```python
from build123d import *

# Parameters (mm, degrees)
SKETCH1_W           = 20
SKETCH1_H           = 18
BOSS_EXTRUDE1_DEPTH = 8
SKETCH2_W           = 18
SKETCH2_H           = 5
CUT_EXTRUDE1_DEPTH  = 6
SKETCH4_W           = 18
SKETCH4_H           = 5
CUT_EXTRUDE2_DEPTH  = 13
SKETCH5_W           = 18
SKETCH5_H           = 4
CUT_EXTRUDE3_DEPTH  = 4


with BuildPart() as part:
    # Sketch1 → Boss-Extrude1 (new body)
    with BuildSketch(Plane.XY):
        Rectangle(SKETCH1_W, SKETCH1_H)
    extrude(amount=BOSS_EXTRUDE1_DEPTH)

    # Sketch2 → Cut-Extrude1 (cut)
    with BuildSketch(Plane.XY.offset(8)):
        with Locations((0, -5.5)):
            Rectangle(SKETCH2_W, SKETCH2_H)
    extrude(amount=-CUT_EXTRUDE1_DEPTH, mode=Mode.SUBTRACT)

    # Sketch4 → Cut-Extrude2 (cut)
    with BuildSketch(Plane.XZ.offset(3)):
        with Locations((0, 4.5)):
            Rectangle(SKETCH4_W, SKETCH4_H)
    extrude(amount=-CUT_EXTRUDE2_DEPTH, mode=Mode.SUBTRACT)

    # Sketch5 → Cut-Extrude3 (cut)
    with BuildSketch(Plane(origin=(0, 0, 0), x_dir=(-1, 0, 0), z_dir=(0, 0, -1))):
        with Locations((0, 7)):
            Rectangle(SKETCH5_W, SKETCH5_H)
    extrude(amount=-CUT_EXTRUDE3_DEPTH, mode=Mode.SUBTRACT)


solid = part.part
```
The model under review builds one solid part; all positions refer to its coordinate system, in mm. A direction names the side the tool comes from. Round coordinates to 2 decimals unless told otherwise and drop trailing zeros. Order: outer loops, then holes, each group sorted by start corner. A loop starts at its lowest first (then second) coordinate and runs counter-clockwise, first axis right, second up.
Item 1: To check wall thickness, follow probe 1 along Z at (x, y) = (-6.25, -2); probe 2 along X at (y, z) = (1, 5.75); probe 3 along Y at (x, z) = (-2.75, 0.75). State the ranges of each line that lie inside material, in increasing order.
Working result:
probe 1: z = 0 to 2, 7 to 8
probe 2: x = -10 to -9, 9 to 10
probe 3: y = -9 to 5
Item 2: For pin 1 (1.8 mm diameter, centred on x = 2, z = 4, fed in from +Y); pin 2 (1 mm diameter, centred on x = 1.5, z = 1, fed in from +Y), all flat-tipped, find the tip position at first contact; note any pin that passes through.
Working result:
pin 1: stops at y = -8
pin 2: stops at y = 5
Item 3: Draft analysis for pull direction X (two halves, no side actions). For faces 5 (the flat face through (0, 2, 8)), 6 (the flat face through (-10, 0, 4)), 7 (the flat face through (-9, 0, 4)), 8 (the flat face through (10, 0, 4)), state which applies: released by +X, released by -X, zero draft, split by the parting line, or undercut.
Working result:
face 5: zero draft
face 6: released by -X
face 7: undercut
face 8: released by +X
Item 4: Add section D-D, the plane y = -5.75. State the section outline as (x, z) points.
Working result:
outline: (-10, 0) - (10, 0) - (10, 8) - (9, 8) - (9, 2) - (-9, 2) - (-9, 8) - (-10, 8) - close
Item 5: Machinability: for faces 1 (the flat face through (0, 5, 1)), 2 (the flat face through (0, -2, 2)), 3 (the flat face through (-0.1, -3, 7.5)), 4 (the flat face through (0, -9, 4)), which of the approach directions +Z, -Z, +X, -X, +Y, -Y give a long, thin tool a straight path to every point of the face, cutting with its end or side? Answer none if there is none.
Working result:
face 1: -Z, +Y
face 2: +Y
face 3: +Z
face 4: +Z, -Z, +X, -X, -Y
Item 6: Add section B-B, the plane x = 5.25. State the section outline as (y, z) points.
Working result:
outline: (-9, 0) - (5, 0) - (5, 2) - (-8, 2) - (-8, 8) - (-9, 8) - close; (-3, 7) - (9, 7) - (9, 8) - (-3, 8) - close
Item 7: Add section A-A, the plane y = -1.75. State the section outline as (x, z) points.
Working result:
outline: (-10, 0) - (10, 0) - (10, 8) - (-10, 8) - close; hole (-9, 2) - (9, 2) - (9, 7) - (-9, 7) - close
Item 8: Add section C-C, the plane z = 4.25. State the section outline as (x, y) points, and give its area (3 significant figures).
Working result:
outline: (-10, -9) - (10, -9) - (10, 9) - (9, 9) - (9, -8) - (-9, -8) - (-9, 9) - (-10, 9) - close
area: 54.0 mm2
